```python
from build123d import *

# Parameters (mm, degrees)
SKIZZE1_R                       = 23
AUFSATZ_LINEAR_AUSTRAGEN1_DEPTH = 5
SKIZZE2_W                       = 5.200502725
SKIZZE2_H                       = 4
SKIZZE2_W_2                     = 4.740793673
AUFSATZ_LINEAR_AUSTRAGEN2_DEPTH = 5
SKIZZE3_W                       = 5.510037568
SKIZZE3_H                       = 140
SKIZZE3_W_2                     = 5.050328516
AUFSATZ_LINEAR_AUSTRAGEN3_DEPTH = 3
SKIZZE4_W                       = 5
SKIZZE4_H                       = 3
AUFSATZ_LINEAR_AUSTRAGEN4_DEPTH = 3
SKIZZE5_W                       = 5
SKIZZE5_H                       = 3
AUFSATZ_LINEAR_AUSTRAGEN5_DEPTH = 3


with BuildPart() as part:
    # Skizze1 → Aufsatz-Linear austragen1 (new body)
    with BuildSketch(Plane.XY):
        with BuildLine():
            Line((64.700502725, 4), (59.190465157, 4))
            ThreePointArc((59.190465157, 4), (34.007664459, 25.995043312), (7.985298356, 5))
            ThreePointArc((7.985298356, 5), (-0.004875067, 9.908732253), (-7.980769231, 4.976832421))
            ThreePointArc((-7.980769231, 4.976832421), (-33.995863589, 25.995271095), (-59.190465157, 4))
            Line((-59.190465157, 4), (-64.240793673, 4))
            Line((-64.240793673, 4), (-64.240793673, 0))
            Line((-64.240793673, 0), (-59.5, 0))
            ThreePointArc((-59.5, 0), (-33.5, -26), (-7.5, 0))
            ThreePointArc((-7.5, 0), (0, 7.5), (7.5, 0))
            ThreePointArc((7.5, 0), (33.5, -26), (59.5, 0))
            Line((59.5, 0), (64.700502725, 0))
            Line((64.700502725, 0), (64.700502725, 4))
        make_face()
        with Locations((33.5, 0)):
            Circle(SKIZZE1_R, mode=Mode.SUBTRACT)
        with Locations((-33.5, 0)):
            Circle(SKIZZE1_R, mode=Mode.SUBTRACT)
    extrude(amount=AUFSATZ_LINEAR_AUSTRAGEN1_DEPTH)

    # Skizze2 → Aufsatz-Linear austragen2 (add)
    with BuildSketch(Plane(origin=(0, 0, 0), x_dir=(-1, 0, 0), z_dir=(0, 0, -1))):
        with Locations((-62.100251363, 2)):
            Rectangle(SKIZZE2_W, SKIZZE2_H)
        with Locations((61.870396837, 2)):
            Rectangle(SKIZZE2_W_2, SKIZZE2_H)
    extrude(amount=AUFSATZ_LINEAR_AUSTRAGEN2_DEPTH)

    # Skizze3 → Aufsatz-Linear austragen3 (add)
    with BuildSketch(Plane(origin=(0, 4, 0), x_dir=(1, 0, 0), z_dir=(0, 1, 0))):
        with Locations((61.945483941, 65)):
            Rectangle(SKIZZE3_W, SKIZZE3_H)
        with Locations((-61.715629415, 65)):
            Rectangle(SKIZZE3_W_2, SKIZZE3_H)
    extrude(amount=AUFSATZ_LINEAR_AUSTRAGEN3_DEPTH)

    # Skizze4 → Aufsatz-Linear austragen4 (add)
    with BuildSketch(Plane.ZY.offset(-59.190465157)):
        with Locations((2.5, 5.5)):
            Rectangle(SKIZZE4_W, SKIZZE4_H)
    extrude(amount=AUFSATZ_LINEAR_AUSTRAGEN4_DEPTH)

    # Skizze5 → Aufsatz-Linear austragen5 (add)
    with BuildSketch(Plane(origin=(-59.190465157, 0, 0), x_dir=(0, 0, -1), z_dir=(1, 0, 0))):
        with Locations((-2.5, 5.5)):
            Rectangle(SKIZZE5_W, SKIZZE5_H)
    extrude(amount=AUFSATZ_LINEAR_AUSTRAGEN5_DEPTH)


solid = part.part
```
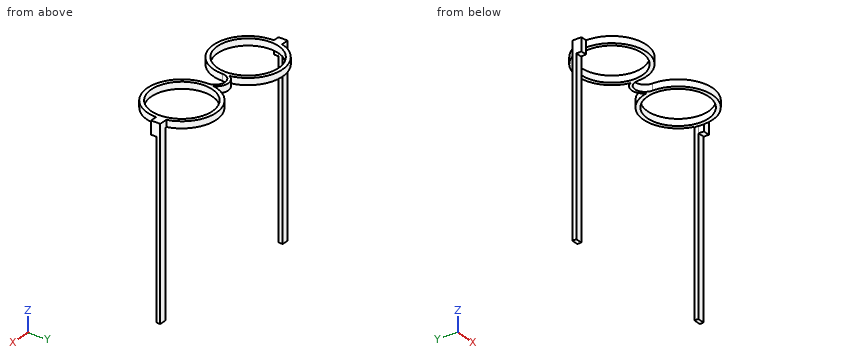
The model under review builds one solid part; all positions refer to its coordinate system, in mm. Round coordinates to 2 decimals unless told otherwise and drop trailing zeros. Order: outer loops, then holes, each group sorted by start corner. A loop starts at its lowest first (then second) coordinate and runs counter-clockwise, first axis right, second up.
Item 1: Add section B-B, the plane z = -47. State the section outline as (x, y) points, and give its area (3 significant figures).
Working result:
outline: (-64.24, 4) - (-59.19, 4) - (-59.19, 7) - (-64.24, 7) - close; (59.19, 4) - (64.7, 4) - (64.7, 7) - (59.19, 7) - close
area: 31.7 mm2
Item 2: Add section D-D, the plane y = 17. State the section outline as (x, z) points, and give its area (3 significant figures).
Working result:
outline: (-53.17, 0) - (-48.99, 0) - (-48.99, 5) - (-53.17, 5) - close; (-18.01, 0) - (-13.83, 0) - (-13.83, 5) - (-18.01, 5) - close; (13.83, 0) - (18.01, 0) - (18.01, 5) - (13.83, 5) - close; (48.99, 0) - (53.17, 0) - (53.17, 5) - (48.99, 5) - close
area: 83.6 mm2
Item 3: For pin 1 (4.5 mm diameter, centred on x = 61, z = -73, fed in from -Y); pin 2 (3 mm diameter, centred on x = -61, z = -79.5, fed in from +Y); pin 3 (8 mm diameter, centred on x = -27.5, y = -14.5, fed in from -Z); pin 4 (5.5 mm diameter, centred on x = 63.5, z = 2.5, fed in from -Y), all flat-tipped, find the tip position at first contact; note any pin that passes through.
Working result:
pin 1: stops at y = 4
pin 2: stops at y = 7
pin 3: passes through
pin 4: stops at y = 0
Item 4: Add section C-C, the plane y = -5. State the section outline as (x, z) points, and give its area (3 significant figures).
Working result:
outline: (-59.01, 0) - (-55.95, 0) - (-55.95, 5) - (-59.01, 5) - close; (-11.05, 0) - (-7.99, 0) - (-7.99, 5) - (-11.05, 5) - close; (7.99, 0) - (11.05, 0) - (11.05, 5) - (7.99, 5) - close; (55.95, 0) - (59.01, 0) - (59.01, 5) - (55.95, 5) - close
area: 61.3 mm2
Item 5: To check wall thickness, follow probe 1 along Y at (x, z) = (33, 2); probe 2 along Z at (x, y) = (43.5, 23). State the ranges of each line that lie inside material, in increasing order.
Working result:
probe 1: y = -26 to -22.99, 22.99 to 26
probe 2: z = 0 to 5
Item 6: Add section A-A, the plane x = 33.5. State the section outline as (y, z) points, and give its area (3 significant figures).
Working result:
outline: (-26, 0) - (-23, 0) - (-23, 5) - (-26, 5) - close; (23, 0) - (26, 0) - (26, 5) - (23, 5) - close
area: 30.0 mm2
